Part model, mm, in its own coordinate system. A direction names the side the tool comes from. Coordinates: 2 decimals unless noted, no trailing zeros. Loops run counter-clockwise (first coordinate to the right, second up) from the corner with the lowest first, then second, coordinate; pieces in that order, holes last. Notation, with made-up numbers: M 46,80.25 L 62,80.25 A20 ccw 62,91.25 Z; hole C 86.25,-19 d9. An arc over 180 degrees is marked long. Use a Markdown table: item, result. Add a question column.
1) Wall check: probe 1 along Y at (x, z) = (-30, 3.9); probe 2 along X at (y, z) = (10, 1.45); probe 3 along X at (y, z) = (-10, 2.2). Give the ranges that are in metal, low to high. Write a range as from..to.
2) Band-saw the part on B-B (z = 14). List the corners of the cut face in (x, y), plus the area to 3 significant figures.
3) Pin check, flat tips, straight feed: pin 1 Ø4.5 at (x, z) = (-37, 3.5) entering from +Y; pin 2 Ø2.5 at (x, y) = (30, -10) entering from +Z; pin 3 Ø4 at (x, z) = (-20.5, 14.5) entering from +Y; pin 4 Ø2.5 at (x, y) = (8.7, 0) entering from -Z. Stop position of each tip, or through.
4) Tool access for faces 4 (the flat face through (35, -13, 4)), 5 (the cylindrical face through (18.4, 7.5, 1)), 6 (the flat face through (-30, -10, 5)): list every direction of +Z, -Z, +X, -X, +Y, -Y with a clear straight run to the whole face (end or side of a thin tool).
5) Pull direction Y, two halves, no side cores. Call faces 1 (the flat face through (36, 7, 4)), 2 (the flat face through (-1, -9, 0)), 3 (the cylindrical face through (-3, 44.9, 10.9)): released by +Y, released by -Y, zero draft, split by the parting line, or undercut.
Autodesk Fusion 360 part; units mm, degrees
sketch "스케치1" plane through (0, 0, 0) normal (0, 0, 1) x (1, 0, 0)
  circle A0 centre (0, 0) radius 45
  dimension "d1" = 90
extrude "돌출1" add sketch "스케치1" along normal blind 2
sketch "스케치2" plane through (0, 0, 2) normal (0, 0, 1) x (-1, 0, 0)
  circle A0 centre (0, 0) radius 45
  circle A1 centre (0, 0) radius 43
  dimension "d4" = 86
  dimension "d5" = 90
extrude "돌출2" add sketch "스케치2" along normal blind 18
fillet "필렛1" radius 2 1 edges at (-41.9547, -16.2727, 0)
sketch "스케치4" plane through (0, 0, 2) normal (0, 0, 1) x (-1, 0, 0)
  circle A0 centre (0, 0) radius 43
  line L0 (-30, -13) -> (-40.9878, -13)
  line L1 (-30, -7) -> (-42.4264, -7)
  line L2 (-30, 7) -> (-42.4264, 7)
  line L3 (-30, 13) -> (-40.9878, 13)
  line L4 (30, -13) -> (40.9878, -13)
  line L5 (30, -7) -> (42.4264, -7)
  line L6 (30, 7) -> (42.4264, 7)
  line L7 (30, 13) -> (40.9878, 13)
  arc A1 (30, 13) -> (30, 7) centre (30, 10) ccw
  arc A2 (30, -7) -> (30, -13) centre (30, -10) ccw
  arc A3 (-30, -13) -> (-30, -7) centre (-30, -10) ccw
  arc A4 (-30, 7) -> (-30, 13) centre (-30, 10) ccw
  dimension "d32" = 6
  dimension "d33" = 60
  dimension "d34" = 20
  dimension "d35" = 10
  dimension "d36" = 30
  dimension "d46" = 6
  dimension "d47" = 6
extrude "돌출7" add sketch "스케치4" along normal blind 5 contours A0 L6 L7 A1 | A0 L4 L5 A2 | A0 L2 L3 A4 | A0 L0 L1 A3
sketch "스케치7" plane through (0, 0, 0) normal (0, 0, -1) x (1, 0, 0)
  arc A0 (-30, -13) -> (-30, -7) centre (-30, -10) ccw construction
  arc A1 (-30, 7) -> (-30, 13) centre (-30, 10) ccw construction
  arc A2 (30, 13) -> (30, 7) centre (30, 10) ccw construction
  arc A3 (30, -7) -> (30, -13) centre (30, -10) ccw construction
  circle A4 centre (-30, 10) radius 1.45
  circle A5 centre (-30, -10) radius 1.45
  circle A6 centre (30, -10) radius 1.45
  circle A7 centre (30, 10) radius 1.45
  dimension "d42" = 2.9
extrude "돌출8" cut sketch "스케치7" against normal blind 5
fillet "필렛2" radius 1 12 edges at (-35.4939, -13, 7) (-27, -10, 7) (-36.2132, -7, 7) (-36.2132, 7, 7) (-27, 10, 7) (-35.4939, 13, 7) (35.4939, 13, 7) (27, 10, 7) (36.2132, 7, 7) (36.2132, -7, 7) (27, -10, 7) (35.4939, -13, 7)
sketch "스케치9" plane through (0, 0, 2) normal (0, 0, 1) x (-1, 0, 0)
  circle A0 centre (0, 0) radius 15
  dimension "d50" = 30
extrude "돌출9" add sketch "스케치9" along normal blind 1
sketch "스케치10" plane through (0, 0, 3) normal (0, 0, 1) x (-1, 0, 0)
  circle A0 centre (0, 0) radius 2
  circle A1 centre (-8.7, 0) radius 2
  circle A2 centre (8.7, 0) radius 2
  dimension "d53" = 8.7
  dimension "d54" = 8.7
  dimension "d55" = 4
extrude "돌출10" cut sketch "스케치10" against normal blind 3
sketch "스케치11" plane through (0, 0, 0) normal (0, 0, -1) x (1, 0, 0)
  line L0 (21, 5) -> (21, -5)
  line L1 (16, -5) -> (16, 5)
  line L2 (-16, 5) -> (-16, -5)
  line L3 (-21, -5) -> (-21, 5)
  arc A0 (-16, 5) -> (-21, 5) centre (-18.5, 5) ccw
  arc A1 (-21, -5) -> (-16, -5) centre (-18.5, -5) ccw
  arc A2 (16, -5) -> (21, -5) centre (18.5, -5) ccw
  arc A3 (21, 5) -> (16, 5) centre (18.5, 5) ccw
  dimension "d58" = 5
  dimension "d60" = 10
  dimension "d61" = 16
  dimension "d62" = 5
  dimension "d63" = 16
  dimension "d64" = 2.5
  dimension "d65" = 5
extrude "돌출11" cut sketch "스케치11" against normal blind 2
Entries:
| question | item | result |
|---|---|---|
| 1 | probe 1 | -33.54..-30.81, -13..-11.45, -8.55..-7, 7..8.55, 11.45..13, 30.81..33.54 |
| 1 | probe 2 | -43.8..-31.45, -28.55..28.55, 31.45..43.8 |
| 1 | probe 3 | -43.87..-31.45, -28.55..-27, -11.18..11.18, 27..28.55, 31.45..43.87 |
| 2 | outline | C 0,0 d90; hole C 0,0 d86 |
| 2 | area | 553 mm2 |
| 3 | pin 1 | y = 28.59 |
| 3 | pin 2 | z = 7 |
| 3 | pin 3 | y = 41.02 |
| 3 | pin 4 | through |
| 4 | face 4 | +Z |
| 4 | face 5 | +Z, -Z |
| 4 | face 6 | -Z |
| 5 | face 1 | undercut |
| 5 | face 2 | zero draft |
| 5 | face 3 | split by the parting line |
